```python
from build123d import *

# Parameters (mm, degrees)
SKETCH2_R           = 4.5
BOSS_EXTRUDE1_DEPTH = 25
BOSS_EXTRUDE2_DEPTH = 5
SKETCH4_R           = 3
CUT_EXTRUDE1_DEPTH  = 20
FILLET1_R           = 10
FILLET3_R           = 1
SKETCH6_R           = 5
CUT_EXTRUDE2_DEPTH  = 20


with BuildPart() as part:
    # Sketch1 → Revolve1 (revolve)
    with BuildSketch(Plane.XY):
        with BuildLine():
            Line((0, 7), (0, -7))
            ThreePointArc((0, -7), (7, 0), (0, 7))
        make_face()
    revolve(axis=Axis((0, 7, 0), (0, -1, 0)))

    # Sketch2 → Boss-Extrude1 (add)
    with BuildSketch(Plane.XY):
        with Locations(Location((0, 0, 0), (0, 0, 180))):
            Circle(SKETCH2_R)
    extrude(amount=BOSS_EXTRUDE1_DEPTH)

    # Sketch3 → Boss-Extrude2 (add)
    with BuildSketch(Plane.XY.offset(25)):
        Polygon((5.687720884, -1.910453125), (4.498361381, 3.970484213), (-1.189359503, 5.880937338), (-5.687720884, 1.910453125), (-4.498361381, -3.970484213), (1.189359503, -5.880937338), align=None)
    extrude(amount=BOSS_EXTRUDE2_DEPTH)

    # Sketch4 → Cut-Extrude1 (cut)
    with BuildSketch(Plane.XY.offset(30)):
        Circle(SKETCH4_R)
    extrude(amount=-CUT_EXTRUDE1_DEPTH, mode=Mode.SUBTRACT)

    # Fillet1
    fillet1_edges = [part.edges().sort_by_distance(p)[0] for p in [
        (4.5, 0, 5.361902647),
    ]]
    fillet(fillet1_edges, radius=FILLET1_R)

    # Fillet3
    fillet3_edges = [part.edges().sort_by_distance(p)[0] for p in [
        (4.5, 0, 25),
    ]]
    fillet(fillet3_edges, radius=FILLET3_R)

    # Sketch5 → Cut-Revolve1 (revolve, cut)
    with BuildSketch(Plane(origin=(0, 0, 0), x_dir=(0, 0, -1), z_dir=(1, 0, 0))):
        with BuildLine():
            Line((6, 0), (-6, 0))
            ThreePointArc((-6, 0), (0, -6), (6, 0))
        make_face()
    revolve(axis=Axis((0, 0, -6), (0, 0, 1)), mode=Mode.SUBTRACT)

    # Sketch6 → Cut-Extrude2 (cut)
    with BuildSketch(Plane(origin=(0, 0, 0), x_dir=(0, 0, -1), z_dir=(1, 0, 0))):
        Circle(SKETCH6_R)
    extrude(amount=-CUT_EXTRUDE2_DEPTH, mode=Mode.SUBTRACT)


solid = part.part
```
The listing builds one solid part. Answer for the finished solid, in the listing's coordinates (mm). A direction names the side the tool comes from. Give positions to 0.01 mm unless a question says otherwise; leave off trailing zeros. Write each loop counter-clockwise with the first axis right and the second up, starting at its lowest first coordinate (ties: lowest second). Pieces come first, ordered by that corner, then holes. Notation, with made-up numbers: (-21, 28.25) -> (28, 28.25) arc R16 cw to (28, 56.25) -> close; hole circle Ø4 at (76.5, 81). An arc over 180 degrees is marked (long way). Use one line per item in the form item = value.
1) Section B-B on z = 0 is taken. Write down the section's boundary in (x, y), plus the area to 3 significant figures.
Result:
outline = (-4.9, -5) arc R7 ccw (long way) to (-4.9, 5) -> (-3.32, 5) arc R6 cw (long way) to (-3.32, -5) -> close
area = 29.4 mm²
2) Section A-A on z = 21.5 is taken. Write down the section's boundary in (x, y).
Result:
outline = circle Ø9 at (0, 0); hole circle Ø6 at (0, 0)
3) A tool of negligible diameter and unlimited length cuts with its end or side. For faces 4 (the flat face through (-5.1, -1, 27.5)), 5 (the flat face through (3.41, -3.92, 27.46)), 6 (the flat face through (-4.3, -3.7, 25)), from which of +Z, -Z, +X, -X, +Y, -Y can it reach the whole face along a straight path? Write none if from no direction.
Result:
face_4 = +Z, -X, -Y
face_5 = +Z, +X, -Y
face_6 = -X, -Y
4) Each of these flat-tipped pins is pushed along its axis until it touches: P1, Ø6, axis at x = -4.5, z = 26, coming from the +Y side; P2, Ø1, axis at x = -2, y = 0, coming from the +Z side; P3, Ø8, axis at x = -4.5, y = 3, coming from the -Z side. Where does it stop, or does it pass through?
Result:
P1 = 5.61
P2 = 10
P3 = -6.86
5) For a pull along Y with two mould halves and no side action, classify faces 1 (the flat face through (0, 0, 10)), 2 (the flat face through (1.694, 4.912, 27.465)), 3 (the flat face through (5.4, -1.8, 25)) as +Y half, -Y half, draft (parallel to the pull), parting line (faces both ways), or undercut.
Result:
face_1 = undercut
face_2 = +Y half
face_3 = draft
6) Straight lines are drawn through the part: probe 1 along Y at (x, z) = (0, 17); probe 2 along Z at (x, y) = (-1.25, 5.25); probe 3 along X at (y, z) = (1, 23). For each, find the intervals that lie inside material, in ascending order.
Result:
probe_1 = -4.5 to -3, 3 to 4.5
probe_2 = -4.46 to -2.62, 2.62 to 4.74, 24.99 to 30
probe_3 = -4.39 to -2.83, 2.83 to 4.39
